Part model, mm, in its own coordinate system. Round coordinates to 2 decimals unless told otherwise and drop trailing zeros. Loops run counter-clockwise (first coordinate to the right, second up) from the corner with the lowest first, then second, coordinate; pieces in that order, holes last.
(1) Flat gauge pins, fed straight in: pin 1 (7 mm diameter, centred on x = 0, y = 138.938, fed in from -Z); pin 2 (8 mm diameter, centred on y = 130, z = 0.5, fed in from +X); pin 3 (2 mm diameter, centred on y = 114, z = 4, fed in from -X); pin 4 (4 mm diameter, centred on y = 126, z = 3.5, fed in from +X). Where does each tip first touch, or does it go through?
(2) Cut at C-C on y = 31.5. List the corners of the cut face in (x, z).
(3) Cut at B-B on z = -5. List the corners of the cut face in (x, y).
(4) Cut at A-A on x = 0. List the corners of the cut face in (y, z), then the cut area to 3 significant figures.
(5) Probe probe 1 along Y at (x, z) = (0, -6.5); probe 2 along X at (y, z) = (85, 0.5); probe 3 along Y at (x, z) = (3, 8). List the from-to ranges inside material, lowest first.
(6) Cut at D-D on x = 8.25. List the corners of the cut face in (y, z), then the cut area to 3 significant figures.
from build123d import *

# Parameters (mm, degrees)
SKETCH1_R               = 9.906
BOSS_EXTRUDE1_DEPTH     = 127
SKETCH2_R               = 9.906
BOSS_EXTRUDE2_DEPTH     = 20.828
SKETCH3_R               = 3.81
CUT_EXTRUDE1_DEPTH      = 15.748
CUT_EXTRUDE1_DEPTH_BACK = 15.748


with BuildPart() as part:
    # Sketch1 → Boss-Extrude1 (new body)
    with BuildSketch(Plane(origin=(0, 0, 0), x_dir=(1, 0, 0), z_dir=(0, 1, 0))):
        Circle(SKETCH1_R)
    extrude(amount=BOSS_EXTRUDE1_DEPTH)

    # Sketch2 → Boss-Extrude2 (add)
    with BuildSketch(Plane(origin=(0, 127, 0), x_dir=(1, 0, 0), z_dir=(0, 1, 0))):
        Circle(SKETCH2_R)
    extrude(amount=BOSS_EXTRUDE2_DEPTH)

    # Sketch3 → Cut-Extrude1 (cut, two sides)
    with BuildSketch(Plane.XY) as cut_extrude1_sk:
        with Locations((0, 138.938)):
            Circle(SKETCH3_R)
    extrude(amount=CUT_EXTRUDE1_DEPTH, mode=Mode.SUBTRACT)
    extrude(cut_extrude1_sk.sketch, amount=-CUT_EXTRUDE1_DEPTH_BACK, mode=Mode.SUBTRACT)


solid = part.part
Final values:
1. pin 1: passes through
1. pin 2: stops at x = 9.91
1. pin 3: stops at x = -9.44
1. pin 4: stops at x = 9.79
2. outline: circle Ø19.81 at (0, 0)
3. outline: (-8.55, 0) - (8.55, 0) - (8.55, 147.83) - (-8.55, 147.83) - close; hole circle Ø7.62 at (0, 138.94)
4. outline: (0, -9.91) - (135.13, -9.91) - (135.13, 9.91) - (0, 9.91) - close; (142.75, -9.91) - (147.83, -9.91) - (147.83, 9.91) - (142.75, 9.91) - close
4. area: 2,780 mm2
5. probe 1: y = 0 to 135.13, 142.75 to 147.83
5. probe 2: x = -9.89 to 9.89
5. probe 3: y = 0 to 136.59, 141.29 to 147.83
6. outline: (0, -5.48) - (147.83, -5.48) - (147.83, 5.48) - (0, 5.48) - close
6. area: 1,620 mm2
